from build123d import *

# Parameters (mm, degrees)
F0_R     = 3.5
F1_DEPTH = 2


with BuildPart() as f1:
    # F0 (on Top) → F1 (new body)
    with BuildSketch(Plane.XY):
        Polygon((125, -10), (125, 10), (99.641016, 10), (-99.641016, 10), (-125, 10), (-125, -10), (-99.641016, -10), (99.641016, -10), align=None)
        Circle(F0_R, mode=Mode.SUBTRACT)
        Polygon((99.641016, 10), (125, 10), (119.641016, 30), align=None)
        Polygon((119.641016, -30), (125, -10), (99.641016, -10), align=None)
        Polygon((-125, 10), (-99.641016, 10), (-119.641016, 30), align=None)
        Polygon((-119.641016, -30), (-99.641016, -10), (-125, -10), align=None)
    extrude(amount=F1_DEPTH)


solid = f1.part
Model file for the job. Use its own axes, mm. A direction names the side the tool comes from. Round coordinates to 2 decimals unless told otherwise and drop trailing zeros. Loops run counter-clockwise (first coordinate to the right, second up) from the corner with the lowest first, then second, coordinate; pieces in that order, holes last.
1. Tool access for faces 5 (the flat face through (109.78, 20.14, 0.99)), 6 (the cylindrical face through (3.233, -1.341, 0.986)), 7 (the flat face through (-109.78, -20.14, 0.99)): list every direction of +Z, -Z, +X, -X, +Y, -Y with a clear straight run to the whole face (end or side of a thin tool).
Check values:
face 5: +Z, -Z, +Y
face 6: +Z, -Z
face 7: +Z, -Z, -Y
2. Drop flat-ended pins along their axis: P1, Ø1, axis at x = 52.5, z = 2, coming from the +Y side; P2, Ø1, axis at x = -63, z = 1, coming from the -Y side. Give the stop position or say it passes through.
Check values:
P1: stops at y = 10
P2: stops at y = -10
3. Band-saw the part on A-A, the plane x = 0. List the corners of the cut face in (y, z).
Check values:
outline: (-10, 0) - (-3.5, 0) - (-3.5, 2) - (-10, 2) - close; (3.5, 0) - (10, 0) - (10, 2) - (3.5, 2) - close
4. Wall check: probe 1 along Y at (x, z) = (0, 1.15); probe 2 along Y at (x, z) = (53, 1.8); probe 3 along X at (y, z) = (-2.5, 1.5). Give the ranges that are in metal, low to high.
Check values:
probe 1: y = -10 to -3.5, 3.5 to 10
probe 2: y = -10 to 10
probe 3: x = -125 to -2.45, 2.45 to 125
5. Mould opens along X. For faces 1 (the flat face through (-122.283, 20.14, 0.986)), 2 (the flat face through (122.36, 19.86, 0.99)), 3 (the flat face through (-2, -6, 2)), 4 (the flat face through (-109.5, 19.86, 0.99)) say: +X half, -X half, draft (parallel to the pull), parting line (faces both ways), or undercut.
Check values:
face 1: -X half
face 2: +X half
face 3: draft
face 4: undercut
6. Band-saw the part on B-B, the plane y = 0. List the corners of the cut face in (x, z), and give its area (3 significant figures).
Check values:
outline: (-125, 0) - (-3.5, 0) - (-3.5, 2) - (-125, 2) - close; (3.5, 0) - (125, 0) - (125, 2) - (3.5, 2) - close
area: 486 mm2
7. Band-saw the part on C-C, the plane z = 0.9. List the corners of the cut face in (x, y).
Check values:
outline: (-125, -10) - (-119.64, -30) - (-99.64, -10) - (99.64, -10) - (119.64, -30) - (125, -10) - (125, 10) - (119.64, 30) - (99.64, 10) - (-99.64, 10) - (-119.64, 30) - (-125, 10) - close; hole circle Ø7 at (0, 0)
